Geometry: final body of the model. Coordinates: model frame, mm. A direction names the side the tool comes from. Round coordinates to 2 decimals unless told otherwise and drop trailing zeros. Order: outer loops, then holes, each group sorted by start corner. A loop starts at its lowest first (then second) coordinate and runs counter-clockwise, first axis right, second up. Notation, with made-up numbers: (-6.75, 16) -> (16.25, 16) arc R24 cw to (16.25, 49) -> close; hole circle Ø7 at (-25, -22.75). An arc over 180 degrees is marked (long way). Put each result on its own line as item: value.
```python
from build123d import *

# Parameters (mm, degrees)
SKETCH50_W          = 419.1
SKETCH50_H          = 101.6
BOSS_EXTRUDE4_DEPTH = 9.525
CUT_EXTRUDE7_REACH  = 217.83
CUT_EXTRUDE8_REACH  = 217.83


with BuildPart() as part:
    # Sketch50 → Boss-Extrude4 (new body)
    with BuildSketch(Plane(origin=(0, 0, 0), x_dir=(1, 0, 0), z_dir=(0, 1, 0))):
        Rectangle(SKETCH50_W, SKETCH50_H)
    extrude(amount=BOSS_EXTRUDE4_DEPTH)

    # Sketch51 → Cut-Extrude7 (cut, up to next)
    with BuildSketch(Plane.XZ, mode=Mode.PRIVATE) as cut_extrude7_sk1:
        with BuildLine():
            Line((152.7175, -12.7), (152.7175, -50.8))
            ThreePointArc((152.7175, -50.8), (144.78, -58.7375), (136.8425, -50.8))
            Line((136.8425, -50.8), (136.8425, -12.7))
            ThreePointArc((136.8425, -12.7), (144.78, -4.7625), (152.7175, -12.7))
        make_face()
    cut_extrude7_tool1 = extrude(cut_extrude7_sk1.sketch, amount=-CUT_EXTRUDE7_REACH, mode=Mode.PRIVATE) & part.part
    # Sketch51 → Cut-Extrude7 (cut, up to next)
    with BuildSketch(Plane.XZ, mode=Mode.PRIVATE) as cut_extrude7_sk2:
        with BuildLine():
            Line((40.3225, -50.8), (40.3225, -12.7))
            ThreePointArc((40.3225, -12.7), (48.26, -4.7625), (56.1975, -12.7))
            Line((56.1975, -12.7), (56.1975, -50.8))
            ThreePointArc((56.1975, -50.8), (48.26, -58.7375), (40.3225, -50.8))
        make_face()
    cut_extrude7_tool2 = extrude(cut_extrude7_sk2.sketch, amount=-CUT_EXTRUDE7_REACH, mode=Mode.PRIVATE) & part.part
    cut_extrude7_1 = cut_extrude7_tool1.solids().sort_by_distance((144.78, 0, -31.75))[0]
    add(cut_extrude7_1, mode=Mode.SUBTRACT)
    cut_extrude7_2 = cut_extrude7_tool2.solids().sort_by_distance((48.26, 0, -31.75))[0]
    add(cut_extrude7_2, mode=Mode.SUBTRACT)
    cut_extrude7 = cut_extrude7_1 + cut_extrude7_2  # Cut-Extrude7 as one shape, for the pattern or mirror that repeats it

    # Mirror4: Cut-Extrude7 across plane
    add(cut_extrude7.mirror(Plane(origin=(0, 0, 0), x_dir=(0, 0, 1), z_dir=(1, 0, 0))), mode=Mode.SUBTRACT)

    # Sketch55 → Cut-Extrude8 (cut, up to next)
    with BuildSketch(Plane.XZ, mode=Mode.PRIVATE) as cut_extrude8_sk1:
        with BuildLine():
            Line((113.792, 34.925), (113.792, -34.925))
            ThreePointArc((113.792, -34.925), (111.125, -37.592), (108.458, -34.925))
            Line((108.458, -34.925), (108.458, 34.925))
            ThreePointArc((108.458, 34.925), (111.125, 37.592), (113.792, 34.925))
        make_face()
    cut_extrude8_tool1 = extrude(cut_extrude8_sk1.sketch, amount=-CUT_EXTRUDE8_REACH, mode=Mode.PRIVATE) & part.part
    add(cut_extrude8_tool1.solids().sort_by_distance((111.125, 0, 0))[0], mode=Mode.SUBTRACT)


solid = part.part
```
1. Contact query for a flat-ended pin moving along its axis: P1, Ø5, axis at x = 43.5, y = 2, coming from the -Z side. Output: stop coordinate, or through.
Ans:
P1: z = -9.49
2. Cut plane C-C on x = 48.26. Return loops of the section in (y, z) (1 decimal).
Ans:
outline: (0, -4.8) -> (9.5, -4.8) -> (9.5, 50.8) -> (0, 50.8) -> close
3. Material intervals for probe 1 along X at (y, z) = (4.25, -22.5); probe 2 along X at (y, z) = (7.25, -40); probe 3 along X at (y, z) = (5.25, 28), sorted ascending.
Ans:
probe 1: -209.55 to -152.72, -136.84 to -56.2, -40.32 to 40.32, 56.2 to 108.46, 113.79 to 136.84, 152.72 to 209.55
probe 2: -209.55 to -152.72, -136.84 to -56.2, -40.32 to 40.32, 56.2 to 136.84, 152.72 to 209.55
probe 3: -209.55 to 108.46, 113.79 to 209.55
4. Draft query along Z for faces 1 (the face through (113.792, 5, 0)), 2 (the face through (48.085, 4.696, -4.764)), 3 (the face through (40.322, 5, -32)). Return one class per face: +Z half, -Z half, draft (parallel to the pull), parting line (faces both ways), or undercut.
Ans:
face 1: undercut
face 2: -Z half
face 3: draft
5. Cut plane B-B on z = -19. State how many separate pieces and enclosed holes the cut face has, and give its area (3 significant figures).
Ans:
separate pieces: 6
enclosed holes: 0
area: 3,340 mm²
6. Set-up query: faces 4 (the face through (-152.718, 5, -31)), 5 (the face through (181, 5, -50.8)). Return all of +Z, -Z, +X, -X, +Y, -Y with unobstructed straight access to the full face (end or side cutting, diameter ignored); none if empty.
Ans:
face 4: -Z, +Y, -Y
face 5: -Z, +X, -X, +Y, -Y
